Design review of the part built by this model. Coordinates are the model's own, in mm. Face numbers are marked on the shaded views. A direction names the side the tool comes from. Give positions to 0.01 mm unless a question says otherwise; leave off trailing zeros. Order: outer loops, then holes, each group sorted by start corner. A loop starts at its lowest first (then second) coordinate and runs counter-clockwise, first axis right, second up. Notation, with made-up numbers: (-34.5, -25.5) -> (23.5, -25.5) arc R34 cw to (23.5, 5.5) -> close; hole circle Ø3 at (60, -24). An arc over 180 degrees is marked (long way). Use a Markdown table: item, result. Add a question column.
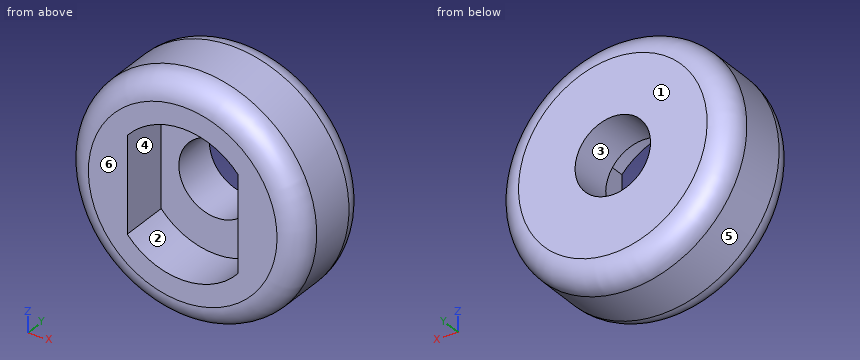
```python
from build123d import *

# Parameters (mm, degrees)
SKETCH_1_R          = 5
SKETCH_1_R_2        = 3.1
SKETCH_1_W          = 4.2
SKETCH_1_H          = 4.5607017
EXTRUDE_1_DEPTH     = 4
SKETCH_2_W          = 4.7
SKETCH_2_H          = 4.043513324
CUT_EXTRUDE_1_DEPTH = 2.1
SKETCH_3_R          = 1.6
CUT_EXTRUDE_2_DEPTH = 3
FILLET_1_R          = 1


with BuildPart() as part:
    # ｽｹｯﾁ1 → ﾎﾞｽ - 押し出し1 (new body)
    # profile 1 of 6: a face of its own
    with BuildSketch(Plane(origin=(0, 0, 0), x_dir=(1, 0, 0), z_dir=(0, 1, 0))):
        with Locations(Location((-75.085298438, 13.647723363, 0), (0, 0, 270))):
            Circle(SKETCH_1_R)
        with Locations((-75.085298438, 13.647723363)):
            Circle(SKETCH_1_R_2, mode=Mode.SUBTRACT)
    # profile 2 of 6: a face of its own
    with BuildSketch(Plane(origin=(0, 0, 0), x_dir=(1, 0, 0), z_dir=(0, 1, 0))):
        with BuildLine():
            ThreePointArc((-71.985298438, 13.647723363), (-72.246284525, 14.892713323), (-72.985298438, 15.928074213))
            Line((-72.985298438, 15.928074213), (-72.985298438, 11.367372513))
            ThreePointArc((-72.985298438, 11.367372513), (-72.246284525, 12.402733403), (-71.985298438, 13.647723363))
        make_face()
    # profile 3 of 6: a face of its own
    with BuildSketch(Plane(origin=(0, 0, 0), x_dir=(1, 0, 0), z_dir=(0, 1, 0))):
        with BuildLine():
            Line((-77.185298438, 11.367372513), (-77.185298438, 15.928074213))
            ThreePointArc((-77.185298438, 15.928074213), (-78.185298438, 13.647723363), (-77.185298438, 11.367372513))
        make_face()
    # profile 4 of 6: a face of its own
    with BuildSketch(Plane(origin=(0, 0, 0), x_dir=(1, 0, 0), z_dir=(0, 1, 0))):
        with BuildLine():
            ThreePointArc((-72.985298438, 15.928074213), (-75.085298438, 16.747723363), (-77.185298438, 15.928074213))
            Line((-77.185298438, 15.928074213), (-72.985298438, 15.928074213))
        make_face()
    # profile 5 of 6: a face of its own
    with BuildSketch(Plane(origin=(0, 0, 0), x_dir=(1, 0, 0), z_dir=(0, 1, 0))):
        with Locations((-75.085298438, 13.647723363)):
            Rectangle(SKETCH_1_W, SKETCH_1_H)
    # profile 6 of 6: a face of its own
    with BuildSketch(Plane(origin=(0, 0, 0), x_dir=(1, 0, 0), z_dir=(0, 1, 0))):
        with BuildLine():
            Line((-72.985298438, 11.367372513), (-77.185298438, 11.367372513))
            ThreePointArc((-77.185298438, 11.367372513), (-75.085298438, 10.547723363), (-72.985298438, 11.367372513))
        make_face()
    extrude(amount=EXTRUDE_1_DEPTH)

    # ｽｹｯﾁ2 → ｶｯﾄ - 押し出し1 (cut)
    with BuildSketch(Plane.XZ):
        with Locations((-75.085298438, -13.647723363)):
            Rectangle(SKETCH_2_W, SKETCH_2_H)
        with BuildLine():
            ThreePointArc((-72.735298438, -11.625966701), (-75.085298438, -10.547723363), (-77.435298438, -11.625966701))
            Line((-77.435298438, -11.625966701), (-72.735298438, -11.625966701))
        make_face()
        with BuildLine():
            Line((-72.735298438, -15.669480025), (-77.435298438, -15.669480025))
            ThreePointArc((-77.435298438, -15.669480025), (-75.085298438, -16.747723363), (-72.735298438, -15.669480025))
        make_face()
    extrude(amount=-CUT_EXTRUDE_1_DEPTH, mode=Mode.SUBTRACT)

    # ｽｹｯﾁ3 → ｶｯﾄ - 押し出し2 (cut)
    with BuildSketch(Plane(origin=(0, 4, 0), x_dir=(1, 0, 0), z_dir=(0, 1, 0))):
        with Locations(Location((-75.085298438, 13.647723363, 0), (0, 0, 270))):
            Circle(SKETCH_3_R)
    extrude(amount=-CUT_EXTRUDE_2_DEPTH, mode=Mode.SUBTRACT)

    # ﾌｨﾚｯﾄ1
    fillet_1_edges = [part.edges().sort_by_distance(p)[0] for p in [
        (-75.085298438, 0, -18.647723363),
        (-75.085298438, 4, -18.647723363),
    ]]
    fillet(fillet_1_edges, radius=FILLET_1_R)


solid = part.part
```
1) Add section A-A (y = 0.7). Give the boundary of the cut face in (x, z).
2) Add section C-C (y = 2.85). Give the boundary of the cut face in (x, z), then the cut area to 3 significant figures.
3) Insertion check: pin 1 (2.5 mm diameter, centred on x = -74.5, z = -14.5, fed in from -Y); pin 2 (0.6 mm diameter, centred on y = 0.5, z = -14, fed in from +X); pin 3 (2 mm diameter, centred on y = 2, z = -15.5, fed in from +X). Each pin has a flat end and moves straight along its axis. Give the tip position at first contact, or say it passes through.
4) The part is to be moulded in two halves that separate along X. For the marked faces 3, 4, 5 and 6, say which applies: +X half, -X half, draft (parallel to the pull), parting line (faces both ways), or undercut.
5) Add section D-D (y = 3.45). Give the boundary of the cut face in (x, z), then the cut area to 3 significant figures.
6) Machinability: for the marked faces 1 and 2, which of the approach directions +Z, -Z, +X, -X, +Y, -Y give a long, thin tool a straight path to every point of the face, cutting with its end or side? Answer none if there is none.
7) For L1, parallel to Z at x = -75.75, y = 0.5; L2, parallel to X at y = 3, z = -13.5; L3, parallel to Z at x = -74.25, y = 2.9, list the stretches that pass through material, from the lowest coordinate up. Write a range as [from, to].
8) Add section B-B (y = 1.55). Give the boundary of the cut face in (x, z), then the cut area to 3 significant figures.
Worked answers:
| question | item | result |
|---|---|---|
| 1 | outline | circle Ø9.91 at (-75.09, -13.65); hole (-77.44, -15.67) arc R3.1 ccw to (-72.74, -15.67) -> (-72.74, -11.63) arc R3.1 ccw to (-77.44, -11.63) -> close |
| 2 | outline | circle Ø10 at (-75.09, -13.65); hole circle Ø3.2 at (-75.09, -13.65) |
| 2 | area | 70.5 mm^2 |
| 3 | pin 1 | y = 2.1 |
| 3 | pin 2 | x = -70.12 |
| 3 | pin 3 | x = -70.16 |
| 4 | face 3 | undercut |
| 4 | face 4 | undercut |
| 4 | face 5 | parting line |
| 4 | face 6 | draft |
| 5 | outline | circle Ø9.79 at (-75.09, -13.65); hole circle Ø3.2 at (-75.09, -13.65) |
| 5 | area | 67.2 mm^2 |
| 6 | face 1 | +Z, -Z, +X, -X, +Y |
| 6 | face 2 | -Y |
| 7 | L1 | [-18.47, -16.68], [-10.62, -8.83] |
| 7 | L2 | [-80.08, -76.68], [-73.49, -70.09] |
| 7 | L3 | [-18.58, -15.01], [-12.28, -8.72] |
| 8 | outline | circle Ø10 at (-75.09, -13.65); hole (-77.44, -15.67) arc R3.1 ccw to (-72.74, -15.67) -> (-72.74, -11.63) arc R3.1 ccw to (-77.44, -11.63) -> close |
| 8 | area | 52.5 mm^2 |
